```python
from build123d import *

# Parameters (mm, degrees)
SKETCH2_W = 1.25
SKETCH2_H = 8
SKETCH4_W = 1.25
SKETCH4_H = 8


with BuildPart() as part:
    # Sketch1 → Revolve1 (revolve)
    with BuildSketch(Plane.XY):
        Polygon((1.451473536, 3), (1.451473536, 7.999829628), (7.451473536, 8), (7.951473536, 8), (7.951473536, 6.325), (14.451473536, 6.325), (14.451473536, 8), (15.451473536, 8), (15.451473536, 3), align=None)
    revolve(axis=Axis((0, 0, 0), (-1, 0, 0)))

    # Sketch2 → M3x0.5 Tapped Hole1 (revolve, cut)
    with BuildSketch(Plane(origin=(3.725736768, 0, 0), x_dir=(0, 0, -1), z_dir=(1, 0, 0))):
        with Locations((0.625, 4)):
            Rectangle(SKETCH2_W, SKETCH2_H)
    revolve(axis=Axis((3.725736768, -6.35, 0), (0, 1, 0)), mode=Mode.SUBTRACT)

    # Sketch4 → M3x0.5 Tapped Hole2 (revolve, cut)
    with BuildSketch(Plane.YZ.offset(3.725736768)):
        with Locations((0.625, 4)):
            Rectangle(SKETCH4_W, SKETCH4_H)
    revolve(axis=Axis((3.725736768, 0, -6.35), (0, 0, 1)), mode=Mode.SUBTRACT)


solid = part.part
```
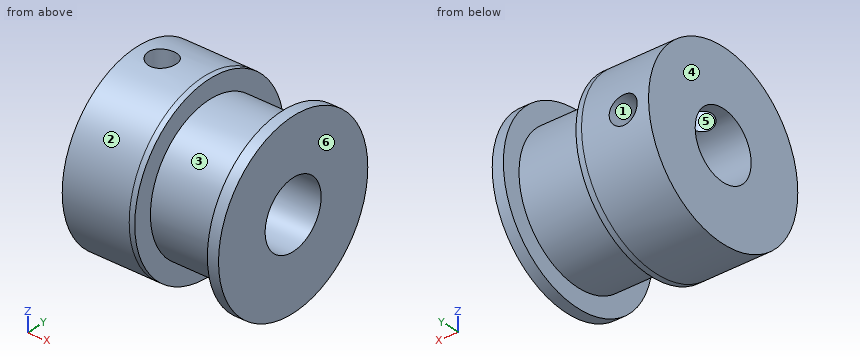
For this review, take the finished solid that the model builds, in its own axes (mm). Face numbers are marked on the shaded views. A direction names the side the tool comes from. Round coordinates to 2 decimals unless told otherwise and drop trailing zeros. Write each loop counter-clockwise with the first axis right and the second up, starting at its lowest first coordinate (ties: lowest second). Pieces come first, ordered by that corner, then holes. Notation, with made-up numbers: M -23,36 L 30,36 A20 cw 30,71 Z; hole C 25.5,17.5 d3. An arc over 180 degrees is marked long. One line per item, written item: value. Start each with the question number.
(1) We need section B-B (z = 2). Give the boundary of the cut face in (x, y), and give its area (3 significant figures).
(2) The part is to be moulded in two halves that separate along X. For the marked faces 4, 5 and 6, say which applies: released by +X, released by -X, zero draft, split by the parting line, or undercut.
(3) Machinability: for the marked faces 1, 2 and 3, which of the approach directions +Z, -Z, +X, -X, +Y, -Y give a long, thin tool a straight path to every point of the face, cutting with its end or side? Answer none if there is none.
(4) Wall thickness on line 1 (X direction, y = 6.75, z = 0); line 2 (Y direction, x = 11.75, z = 0) (3 decimals); line 3 (X direction, y = 6.5, z = 3.75): over which ranges is each line inside the solid? List them lowest first.
(5) We need section C-C (z = 4). Give the boundary of the cut face in (x, y), and give its area (3 significant figures).
(6) We need section A-A (y = 0). Give the boundary of the cut face in (x, z) (3 decimals), and give its area (3 significant figures).
(7) We need section D-D (x = 7). Give the boundary of the cut face in (y, z).
(8) Insertion check: pin 1 (2 mm diameter, centred on x = 9.5, y = 0, fed in from +Z) (3 decimals); pin 2 (2 mm diameter, centred on x = 5.5, y = -5, fed in from +Z); pin 3 (1.5 mm diameter, centred on x = 3.73, z = 0, fed in from +Y). Each pin has a flat end and moves straight along its axis. Give the tip position at first contact, or say it passes through.
Result:
1. outline: M 1.45,-7.75 L 7.95,-7.75 L 7.95,-6 L 14.45,-6 L 14.45,-7.75 L 15.45,-7.75 L 15.45,-2.24 L 1.45,-2.24 Z; M 1.45,2.24 L 15.45,2.24 L 15.45,7.75 L 14.45,7.75 L 14.45,6 L 7.95,6 L 7.95,7.75 L 1.45,7.75 Z
1. area: 132 mm²
2. face 4: released by -X
2. face 5: undercut
2. face 6: released by +X
3. face 1: +Y
3. face 2: +X, -X
3. face 3: none
4. line 1: 1.45 to 2.48, 4.98 to 7.95, 14.45 to 15.45
4. line 2: -6.325 to -3, 3 to 6.325
4. line 3: 1.45 to 7.95, 14.45 to 15.45
5. outline: M 1.45,-6.93 L 7.95,-6.93 L 7.95,-4.9 L 14.45,-4.9 L 14.45,-6.93 L 15.45,-6.93 L 15.45,6.93 L 14.45,6.93 L 14.45,4.9 L 7.95,4.9 L 7.95,6.93 L 1.45,6.93 Z; hole C 3.73,0 d2.5
5. area: 163 mm²
6. outline: M 1.451,-8 L 7.951,-8 L 7.951,-6.325 L 14.451,-6.325 L 14.451,-8 L 15.451,-8 L 15.451,-3 L 1.451,-3 Z; M 1.451,3 L 2.476,3 L 2.476,8 L 1.451,8 Z; M 4.976,3 L 15.451,3 L 15.451,8 L 14.451,8 L 14.451,6.325 L 7.951,6.325 L 7.951,8 L 4.976,8 Z
6. area: 106 mm²
7. outline: C 0,0 d16; hole C 0,0 d6
8. pin 1: z = 6.325
8. pin 2: z = 6.93
8. pin 3: y = -2.9
